Input: part model. Units: mm. Frame: model coordinates. Give positions to 0.01 mm unless a question says otherwise; leave off trailing zeros. Write each loop counter-clockwise with the first axis right and the second up, starting at its lowest first coordinate (ties: lowest second). Pieces come first, ordered by that corner, then holes.
```python
from build123d import *

# Parameters (mm, degrees)
DODANIE_WYCI_GNI_CIE1_DEPTH = 6
SFAZOWANIE1_SIZE            = 5
WYTNIJ_WYCI_GNI_CIE1_REACH  = 258.105
WYTNIJ_WYCI_GNI_CIE2_REACH  = 258.105
SZKIC5_W                    = 6
SZKIC5_H                    = 9
DODANIE_WYCI_GNI_CIE3_DEPTH = 6
WYTNIJ_WYCI_GNI_CIE3_REACH  = 258.105


with BuildPart() as part:
    # Szkic1 → Dodanie-wyciągnięcie1 (new body)
    with BuildSketch(Plane.XY):
        Polygon((0, -185), (0, 185), (25, 185), (177, -135), (177, -185), align=None)
    extrude(amount=DODANIE_WYCI_GNI_CIE1_DEPTH)

    # Sfazowanie1
    sfazowanie1_edges = [part.edges().sort_by_distance(p)[0] for p in [
        (177, -185, 3),
    ]]
    chamfer(sfazowanie1_edges, length=SFAZOWANIE1_SIZE)

    # Szkic2 → Wytnij-wyciągnięcie1 (cut, up to next)
    with BuildSketch(Plane.XY.offset(6), mode=Mode.PRIVATE) as wytnij_wyci_gni_cie1_sk1:
        Polygon((0, -183), (150, -183), (152, -185), (0, -185), align=None)
    wytnij_wyci_gni_cie1_tool1 = extrude(wytnij_wyci_gni_cie1_sk1.sketch, amount=-WYTNIJ_WYCI_GNI_CIE1_REACH, mode=Mode.PRIVATE) & part.part
    add(wytnij_wyci_gni_cie1_tool1.solids().sort_by_distance((75.501104, -184.002208, 6))[0], mode=Mode.SUBTRACT)

    # Szkic3 → Wytnij-wyciągnięcie2 (cut, up to next)
    with BuildSketch(Plane.XY.offset(6), mode=Mode.PRIVATE) as wytnij_wyci_gni_cie2_sk1:
        with BuildLine():
            Line((177, -145), (103.309475019, -145))
            ThreePointArc((103.309475019, -145), (89.5, -150.5), (103.309475019, -156))
            Line((103.309475019, -156), (177, -156))
            Line((177, -156), (177, -145))
        make_face()
    wytnij_wyci_gni_cie2_tool1 = extrude(wytnij_wyci_gni_cie2_sk1.sketch, amount=-WYTNIJ_WYCI_GNI_CIE2_REACH, mode=Mode.PRIVATE) & part.part
    add(wytnij_wyci_gni_cie2_tool1.solids().sort_by_distance((132.134709, -150.5, 6))[0], mode=Mode.SUBTRACT)

    # Szkic5 → Dodanie-wyciągnięcie3 (add)
    with BuildSketch(Plane.ZY):
        with Locations((3, 171.5)):
            Rectangle(SZKIC5_W, SZKIC5_H)
        with Locations((3, 139.5)):
            Rectangle(SZKIC5_W, SZKIC5_H)
        with Locations((3, -144.5)):
            Rectangle(SZKIC5_W, SZKIC5_H)
        with Locations((3, -15.5)):
            Rectangle(SZKIC5_W, SZKIC5_H)
        with Locations((3, 16.5)):
            Rectangle(SZKIC5_W, SZKIC5_H)
    extrude(amount=DODANIE_WYCI_GNI_CIE3_DEPTH)

    # Szkic6 → Wytnij-wyciągnięcie3 (cut, up to next)
    with BuildSketch(Plane.XY.offset(6), mode=Mode.PRIVATE) as wytnij_wyci_gni_cie3_sk1:
        Polygon((12, -156), (12, -158), (0, -158), (0, -160.5), (0, -163), (12, -163), (12, -165), (17, -165), (17, -163), (20, -163), (20, -158), (17, -158), (17, -156), align=None)
    wytnij_wyci_gni_cie3_tool1 = extrude(wytnij_wyci_gni_cie3_sk1.sketch, amount=-WYTNIJ_WYCI_GNI_CIE3_REACH, mode=Mode.PRIVATE) & part.part
    # Szkic6 → Wytnij-wyciągnięcie3 (cut, up to next)
    with BuildSketch(Plane.XY.offset(6), mode=Mode.PRIVATE) as wytnij_wyci_gni_cie3_sk2:
        Polygon((12, 3), (0, 3), (0, -2), (12, -2), (12, -4), (17, -4), (17, -2), (20, -2), (20, 3), (17, 3), (17, 5), (12, 5), align=None)
    wytnij_wyci_gni_cie3_tool2 = extrude(wytnij_wyci_gni_cie3_sk2.sketch, amount=-WYTNIJ_WYCI_GNI_CIE3_REACH, mode=Mode.PRIVATE) & part.part
    # Szkic6 → Wytnij-wyciągnięcie3 (cut, up to next)
    with BuildSketch(Plane.XY.offset(6), mode=Mode.PRIVATE) as wytnij_wyci_gni_cie3_sk3:
        Polygon((12, 158), (0, 158), (0, 153), (12, 153), (12, 151), (17, 151), (17, 153), (20, 153), (20, 158), (17, 158), (17, 160), (12, 160), align=None)
    wytnij_wyci_gni_cie3_tool3 = extrude(wytnij_wyci_gni_cie3_sk3.sketch, amount=-WYTNIJ_WYCI_GNI_CIE3_REACH, mode=Mode.PRIVATE) & part.part
    add(wytnij_wyci_gni_cie3_tool1.solids().sort_by_distance((10.75, -160.5, 6))[0], mode=Mode.SUBTRACT)
    add(wytnij_wyci_gni_cie3_tool2.solids().sort_by_distance((10.75, 0.5, 6))[0], mode=Mode.SUBTRACT)
    add(wytnij_wyci_gni_cie3_tool3.solids().sort_by_distance((10.75, 155.5, 6))[0], mode=Mode.SUBTRACT)


solid = part.part
```
Q1. Section D-D, the plane x = 43. Return the cut outline in (y, z).
Q2. Section B-B, the plane y = -109. Return the cut outline in (x, z).
Q3. Mould query, pull axis X, two halves, no side actions, for faces 1 (the flat face through (66, -39, 0)), 2 (the cylindrical face through (89.504, -150.233, 3.042)), 3 (the flat face through (99.936, 27.24, 2.958)). Classes: +X half, -X half, draft (parallel to the pull), parting line (faces both ways), or undercut.
Q4. Section C-C, the plane x = 134.5. Return the cut outline in (y, z), then the cut area to 3 significant figures.
Q5. Section A-A, the plane x = 97.5. Return the cut outline in (y, z), then the cut area to 3 significant figures.
Q6. Pin query (flat end, axial travel): pin 1 (1 mm diameter, centred on y = -157.5, z = 4.5, fed in from -X); pin 2 (3 mm diameter, centred on x = -2.5, z = 2.5, fed in from -Y); pin 3 (0.6 mm diameter, centred on y = 4, z = 4, fed in from +X). Return the tip coordinate at first contact, or that it passes through.
Q7. Material intervals for line 1 along Y through (x, z) = (14, 4.5); line 2 along X through (y, z) = (-150.5, 3.3); line 3 along Y through (x, z) = (113, 3), sorted ascending.
Solutions:
1. outline: (-183, 0) - (147.11, 0) - (147.11, 6) - (-183, 6) - close
2. outline: (0, 0) - (164.65, 0) - (164.65, 6) - (0, 6) - close
3. face 1: draft
3. face 2: undercut
3. face 3: +X half
4. outline: (-183, 0) - (-156, 0) - (-156, 6) - (-183, 6) - close; (-145, 0) - (-45.53, 0) - (-45.53, 6) - (-145, 6) - close
4. area: 759 mm2
5. outline: (-183, 0) - (-158.5, 0) - (-158.5, 6) - (-183, 6) - close; (-142.5, 0) - (32.37, 0) - (32.37, 6) - (-142.5, 6) - close
5. area: 1,200 mm2
6. pin 1: stops at x = 0
6. pin 2: stops at y = -149
6. pin 3: stops at x = 111.12
7. line 1: y = -183 to -165, -156 to -4, 5 to 151, 160 to 185
7. line 2: x = 0 to 89.5
7. line 3: y = -183 to -156, -145 to -0.26
